Design review of the part built by this model. Coordinates are the model's own, in mm. A direction names the side the tool comes from. Coordinates: 2 decimals unless noted, no trailing zeros. Loops run counter-clockwise (first coordinate to the right, second up) from the corner with the lowest first, then second, coordinate; pieces in that order, holes last. Notation, with made-up numbers: M 56,1 L 95,1 A7 ccw 95,6 Z; hole C 72.5,25 d4. An arc over 180 degrees is marked long. Put each result on its own line as item: value. Start each with the question number.
(1) For probe 1 along Y at (x, z) = (-53.7, 1.45); probe 2 along X at (y, z) = (1.5, 1.6); probe 3 along Y at (x, z) = (63.5, 1.1), list the stretches that pass through material, from the lowest coordinate up. Write a range as [from, to].
(2) Take a section at D-D, the plane z = 1.8. Count the separate pieces of the cut face and the enclosed holes in it, then the cut area to 3 significant figures.
(3) Take a section at C-C, the plane x = 54.5. Give the boundary of the cut face in (y, z).
(4) Take a section at B-B, the plane x = -53.7. Give the boundary of the cut face in (y, z).
(5) Clearance check with flat-ended pins moving along their axes: pin 1 (1.5 mm diameter, centred on y = -17, z = 2, fed in from +X); pin 2 (0.9 mm diameter, centred on x = -60, z = 1.5, fed in from -Y). State where each tip first meets the part, or that it passes through.
(6) Take a section at A-A, the plane y = 0. Give the boundary of the cut face in (x, z).
(7) For faces 1 (the flat face through (18.9, -16, 1)), 2 (the flat face through (-83, -15, 1)), 3 (the cylindrical face through (-58.319, -1.915, 1.479)), list the 3-axis set-ups (+Z, -Z, +X, -X, +Y, -Y) from which the entire face can be reached by the end or side of a thin tool; tool diameter is ignored.
(8) The part is to be moulded in two halves that separate along X. For faces 4 (the flat face through (3.9, -16, 1)), 5 (the flat face through (57, -15, 1)), 6 (the flat face through (23, -18, 2)), say which applies: +X half, -X half, draft (parallel to the pull), parting line (faces both ways), or undercut.
```python
from build123d import *

# Parameters (mm, degrees)
SKETCH1_W           = 187.4
SKETCH1_H           = 30
BOSS_EXTRUDE1_DEPTH = 3
SKETCH2_W           = 7.8
SKETCH2_H           = 3
BOSS_EXTRUDE2_DEPTH = 3
LPATTERN2_COUNT     = 4
LPATTERN2_PITCH     = 22.8
LPATTERN2_COL_COUNT = 4
LPATTERN2_COL_PITCH = 22.8
SKETCH3_R           = 5
CUT_EXTRUDE1_DEPTH  = 96.460410642


with BuildPart() as part:
    # Sketch1 → Boss-Extrude1 (new body)
    with BuildSketch(Plane.XY):
        Rectangle(SKETCH1_W, SKETCH1_H)
    extrude(amount=BOSS_EXTRUDE1_DEPTH)

    # Sketch2 → Boss-Extrude2 (add)
    with BuildSketch(Plane.XZ.offset(15)):
        with Locations((0, 1.5)):
            Rectangle(SKETCH2_W, SKETCH2_H)
    boss_extrude2 = extrude(amount=BOSS_EXTRUDE2_DEPTH)

    # LPattern2: Boss-Extrude2 ×4
    with Locations(*[(i * LPATTERN2_PITCH, 0, 0) for i in range(1, LPATTERN2_COUNT)]):
        add(boss_extrude2)

    # LPattern2 col: Boss-Extrude2 ×4
    with Locations(*[(-i * LPATTERN2_COL_PITCH, 0, 0) for i in range(1, LPATTERN2_COL_COUNT)]):
        add(boss_extrude2)

    # Sketch3 → Cut-Extrude1 (cut, through all)
    with BuildSketch(Plane(origin=(0, 0, 0), x_dir=(-1, 0, 0), z_dir=(0, 0, -1))):
        Circle(SKETCH3_R)
        with Locations((-53.7, 0)):
            Circle(SKETCH3_R)
        with Locations((53.7, 0)):
            Circle(SKETCH3_R)
    extrude(amount=-CUT_EXTRUDE1_DEPTH, mode=Mode.SUBTRACT)


solid = part.part
```
Computed values:
1. probe 1: y = [-15, -5], [5, 15]
1. probe 2: x = [-93.7, -58.47], [-48.93, -4.77], [4.77, 48.93], [58.47, 93.7]
1. probe 3: y = [-15, 15]
2. separate pieces: 1
2. enclosed holes: 3
2. area: 5,550 mm^2
3. outline: M -15,0 L -4.94,0 L -4.94,3 L -15,3 Z; M 4.94,0 L 15,0 L 15,3 L 4.94,3 Z
4. outline: M -15,0 L -5,0 L -5,3 L -15,3 Z; M 5,0 L 15,0 L 15,3 L 5,3 Z
5. pin 1: stops at x = 72.3
5. pin 2: stops at y = -15
6. outline: M -93.7,0 L -58.7,0 L -58.7,3 L -93.7,3 Z; M -48.7,0 L -5,0 L -5,3 L -48.7,3 Z; M 5,0 L 48.7,0 L 48.7,3 L 5,3 Z; M 58.7,0 L 93.7,0 L 93.7,3 L 58.7,3 Z
7. face 1: +Z, -Z, -Y
7. face 2: +Z, -Z, -X, -Y
7. face 3: +Z, -Z
8. face 4: undercut
8. face 5: undercut
8. face 6: draft
